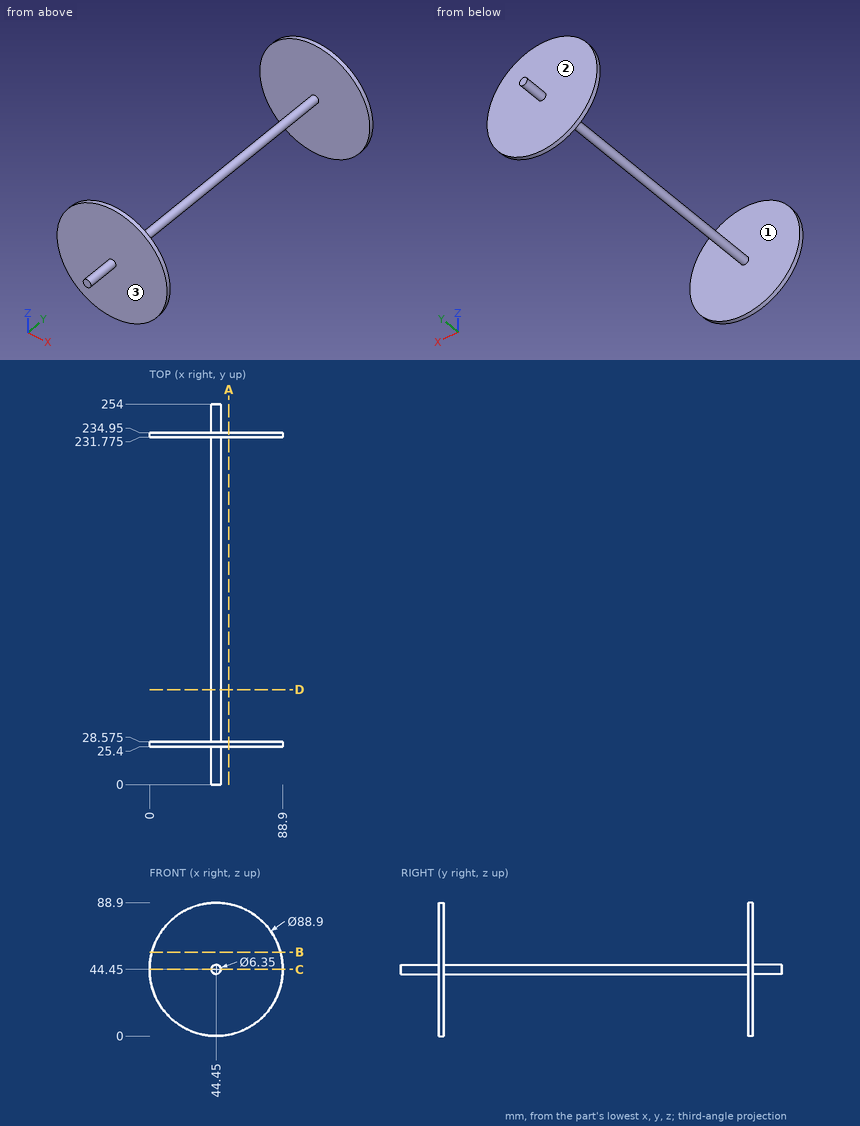
Source: three-view drawing plus pictorial views. Frame: mm from the lowest corner of the part. Round coordinates to 2 decimals unless told otherwise and drop trailing zeros. Order: outer loops, then holes, each group sorted by start corner. A loop starts at its lowest first (then second) coordinate and runs counter-clockwise, first axis right, second up. Notation, with made-up numbers: (72.5, -8) - (115.5, -8) arc R17 cw to (115.5, 16) - close; hole circle Ø8 at (16, -26.5). An arc over 180 degrees is marked (long way). Use a Markdown table: item, result.
1. Section D-D on y = 63.5. Return the cut outline in (x, z) (3 decimals), then the cut area to 3 significant figures.
Evaluation:
| item | result |
|---|---|
| outline | circle Ø6.35 at (44.45, 44.45) |
| area | 31.7 mm^2 |
2. Section B-B on z = 56. Return the cut outline in (x, y) (3 decimals).
Evaluation:
| item | result |
|---|---|
| outline | (1.527, 25.4) - (87.373, 25.4) - (87.373, 28.575) - (1.527, 28.575) - close; (1.527, 231.775) - (87.373, 231.775) - (87.373, 234.95) - (1.527, 234.95) - close |
3. Section A-A on x = 53. Return the cut outline in (y, z) (3 decimals).
Evaluation:
| item | result |
|---|---|
| outline | (25.4, 0.83) - (28.575, 0.83) - (28.575, 88.07) - (25.4, 88.07) - close; (231.775, 0.83) - (234.95, 0.83) - (234.95, 88.07) - (231.775, 88.07) - close |
4. Section C-C on z = 44.45. Return the cut outline in (x, y) (3 decimals), then the cut area to 3 significant figures.
Evaluation:
| item | result |
|---|---|
| outline | (0, 25.4) - (41.275, 25.4) - (41.275, 0) - (47.625, 0) - (47.625, 25.4) - (88.9, 25.4) - (88.9, 28.575) - (47.625, 28.575) - (47.625, 231.775) - (88.9, 231.775) - (88.9, 234.95) - (47.625, 234.95) - (47.625, 254) - (41.275, 254) - (41.275, 234.95) - (0, 234.95) - (0, 231.775) - (41.275, 231.775) - (41.275, 28.575) - (0, 28.575) - close |
| area | 2,140 mm^2 |
5. Mould query, pull axis Y, two halves, no side actions, for the marked faces 1, 2 and 3. Classes: +Y half, -Y half, draft (parallel to the pull), parting line (faces both ways), or undercut.
Evaluation:
| item | result |
|---|---|
| face 1 | undercut |
| face 2 | +Y half |
| face 3 | -Y half |
6. Material intervals for probe 1 along Y at (x, z) = (44, 68) (3 decimals); probe 2 along Z at (x, y) = (79, 233), sorted ascending.
Evaluation:
| item | result |
|---|---|
| probe 1 | 25.4 to 28.575, 231.775 to 234.95 |
| probe 2 | 16.48 to 72.42 |
7. First-contact query: pin 1 (5 mm diameter, centred on x = 41, y = 103, fed in from +Z); pin 2 (2 mm diameter, centred on x = 40, z = 45, fed in from -Y); pin 3 (12 mm diameter, centred on x = 45, y = 127, fed in from -Z) (3 decimals); pin 4 (3 mm diameter, centred on x = 76.5, z = 78.5, fed in from +Y). Flat tips, straight axial feed; report the tip coordinate or a pass-through.
Evaluation:
| item | result |
|---|---|
| pin 1 | z = 47.48 |
| pin 2 | y = 25.4 |
| pin 3 | z = 41.275 |
| pin 4 | through |
